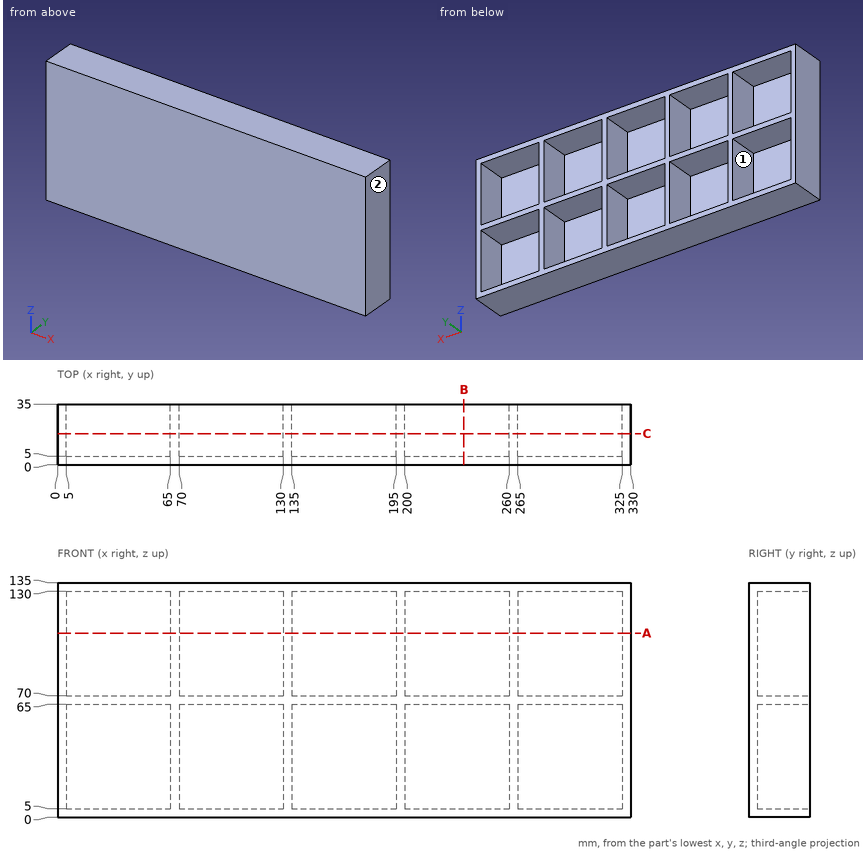
Geometry check sheet. Reference: drawing and pictorial views, mm from the part's lowest x, y, z. Coordinates: 2 decimals unless noted, no trailing zeros. Order: outer loops, then holes, each group sorted by start corner. A loop starts at its lowest first (then second) coordinate and runs counter-clockwise, first axis right, second up. Notation, with made-up numbers: M 40,-37 L 52,-37 A28 cw 52,-15 Z; hole C 78.25,-37.75 d10. An arc over 180 degrees is marked long. Write each question's results on one line, items separated by ' | '. Start each with the question number.
1. Cross-section at A-A on z = 106. Record the cut outline in (x, y).
2. Mould release check, pull along X, two halves, no side actions. Record for the marked faces 1 and 2: +X half, -X half, draft (parallel to the pull), parting line (faces both ways), or undercut.
3. Cross-section at B-B on x = 234. Record the cut outline in (y, z).
4. Material ranges on probe 1 along Z at (x, y) = (38, 8.5); probe 2 along X at (y, z) = (27, 15); probe 3 along Y at (x, z) = (118.5, 20), recorded low to high.
5. Cross-section at C-C on y = 18. State how many separate pieces and enclosed holes the cut face has, and give its area (3 significant figures).
6. Go/stop test with a flat-tipped pin: P1, Ø18, axis at x = 151, z = 113.5, coming from the +Y side. Record where the tip stops, or that it passes through.
Checks:
1) outline: M 0,0 L 330,0 L 330,35 L 325,35 L 325,5 L 265,5 L 265,35 L 260,35 L 260,5 L 200,5 L 200,35 L 195,35 L 195,5 L 135,5 L 135,35 L 130,35 L 130,5 L 70,5 L 70,35 L 65,35 L 65,5 L 5,5 L 5,35 L 0,35 Z
2) face 1: undercut | face 2: +X half
3) outline: M 0,0 L 35,0 L 35,5 L 5,5 L 5,65 L 35,65 L 35,70 L 5,70 L 5,130 L 35,130 L 35,135 L 0,135 Z
4) probe 1: z = 0 to 5, 65 to 70, 130 to 135 | probe 2: x = 0 to 5, 65 to 70, 130 to 135, 195 to 200, 260 to 265, 325 to 330 | probe 3: y = 0 to 5
5) separate pieces: 1 | enclosed holes: 10 | area: 8,550 mm²
6) P1: stops at y = 5
